Geometry check sheet. Reference: the model listing, model coordinates, mm. Face numbers are marked on the shaded views. A direction names the side the tool comes from. Round coordinates to 2 decimals unless told otherwise and drop trailing zeros. Loops run counter-clockwise (first coordinate to the right, second up) from the corner with the lowest first, then second, coordinate; pieces in that order, holes last. Notation, with made-up numbers: (-1.5, -1) -> (3.5, -1) arc R20 cw to (3.5, 14) -> close; hole circle Ø1 at (-10.5, 9.25). An arc over 180 degrees is marked (long way). Use a Markdown table: item, result. Add a question column.
Q1. Release check for a two-part mould opening along X. For the marked faces 3, 4 and 5 record: released by +X, released by -X, zero draft, split by the parting line, or undercut.
Q2. Sectioned sample at B-B, the plane z = 25.5. Enter the section's corners in (x, y).
Q3. Material ranges on L1, parallel to X at y = -10.5, z = 12; L2, parallel to Z at x = 5.5, y = -5.5; L3, parallel to Y at x = 18.25, z = 25.5, recorded low to high.
Q4. Gauge pin test, flat ends, axial feed: P1, Ø1.5, axis at x = 7.5, y = -12.5, coming from the +Z side; P2, Ø2.5, axis at x = 8.8, y = -6.51, coming from the +Z side; P3, Ø4, axis at y = -6.51, z = 25, coming from the +X side. Record the tip position at first contact, or that the pin passes through.
Q5. Sectioned sample at A-A, the plane z = 19. Enter the section's corners in (x, y).
Q6. Set-up check for the marked faces 1 and 2: record each of +Z, -Z, +X, -X, +Y, -Y from which the full face is reachable in a straight line by a thin tool's end or side.
Q7. Sectioned sample at C-C, the plane y = -8.5. Enter the section's corners in (x, z).
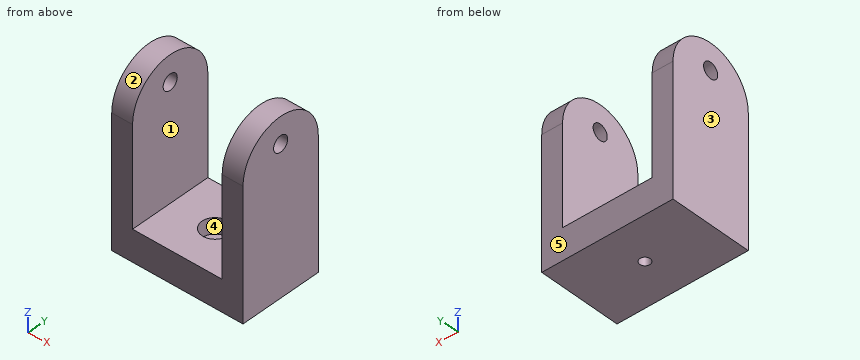
```python
from build123d import *

# Parameters (mm, degrees)
IZIM1_W                     = 25.2
IZIM1_H                     = 16
Y_KSEKLIK_EKSTR_ZYON1_DEPTH = 3
IZIM3_W                     = 4
IZIM3_H                     = 16
Y_KSEKLIK_EKSTR_ZYON2_DEPTH = 30
KES_EKSTR_ZYON3_DEPTH       = 30
IZIM5_R                     = 1.5
KES_EKSTR_ZYON4_DEPTH       = 30
IZIM6_R                     = 2.5
KES_EKSTR_ZYON5_DEPTH       = 4
IZIM7_R                     = 1
KES_EKSTR_ZYON6_DEPTH       = 15


with BuildPart() as part:
    # Çizim1 → Yükseklik-Ekstrüzyon1 (new, symmetric)
    with BuildSketch(Plane.XY):
        with Locations((8.796736324, -6.511156057)):
            Rectangle(IZIM1_W, IZIM1_H)
    extrude(amount=Y_KSEKLIK_EKSTR_ZYON1_DEPTH, both=True)

    # Çizim3 → Yükseklik-Ekstrüzyon2 (add)
    with BuildSketch(Plane.XY):
        with Locations((-1.803263676, -6.511156057)):
            Rectangle(IZIM3_W, IZIM3_H)
        with Locations((19.396736324, -6.511156057)):
            Rectangle(IZIM3_W, IZIM3_H)
    extrude(amount=Y_KSEKLIK_EKSTR_ZYON2_DEPTH)

    # Çizim4 → Kes-Ekstrüzyon3 (cut, symmetric)
    with BuildSketch(Plane(origin=(0, 0, 0), x_dir=(0, 0, -1), z_dir=(1, 0, 0))):
        with BuildLine():
            Line((-22, 1.488843943), (-31.468609906, 1.488843943))
            Line((-31.468609906, 1.488843943), (-31.468609906, -14.511156057))
            Line((-31.468609906, -14.511156057), (-22, -14.511156057))
            ThreePointArc((-22, -14.511156057), (-30, -6.511156057), (-22, 1.488843943))
        make_face()
    extrude(amount=KES_EKSTR_ZYON3_DEPTH, both=True, mode=Mode.SUBTRACT)

    # Çizim5 → Kes-Ekstrüzyon4 (cut, symmetric)
    with BuildSketch(Plane(origin=(0, 0, 0), x_dir=(0, 0, -1), z_dir=(1, 0, 0))):
        with Locations(Location((-25, -6.511156057, 0), (0, 0, 90))):
            Circle(IZIM5_R)
    extrude(amount=KES_EKSTR_ZYON4_DEPTH, both=True, mode=Mode.SUBTRACT)

    # Çizim6 → Kes-Ekstrüzyon5 (cut)
    with BuildSketch(Plane.XY):
        with Locations((8.796736324, -6.511156057)):
            Circle(IZIM6_R)
    extrude(amount=KES_EKSTR_ZYON5_DEPTH, mode=Mode.SUBTRACT)

    # Çizim7 → Kes-Ekstrüzyon6 (cut)
    with BuildSketch(Plane.XY):
        with Locations((8.796736324, -6.511156057)):
            Circle(IZIM7_R)
    extrude(amount=-KES_EKSTR_ZYON6_DEPTH, mode=Mode.SUBTRACT)


solid = part.part
```
Values:
| question | item | result |
|---|---|---|
| 1 | face 3 | released by -X |
| 1 | face 4 | undercut |
| 1 | face 5 | zero draft |
| 2 | outline | (-3.8, -13.7) -> (0.2, -13.7) -> (0.2, -7.93) -> (-3.8, -7.93) -> close; (-3.8, -5.1) -> (0.2, -5.1) -> (0.2, 0.68) -> (-3.8, 0.68) -> close; (17.4, -13.7) -> (21.4, -13.7) -> (21.4, -7.93) -> (17.4, -7.93) -> close; (17.4, -5.1) -> (21.4, -5.1) -> (21.4, 0.68) -> (17.4, 0.68) -> close |
| 3 | L1 | -3.8 to 0.2, 17.4 to 21.4 |
| 3 | L2 | -3 to 3 |
| 3 | L3 | -13.7 to -7.93, -5.1 to 0.68 |
| 4 | P1 | z = 3 |
| 4 | P2 | z = 0 |
| 4 | P3 | x = 21.4 |
| 5 | outline | (-3.8, -14.51) -> (0.2, -14.51) -> (0.2, 1.49) -> (-3.8, 1.49) -> close; (17.4, -14.51) -> (21.4, -14.51) -> (21.4, 1.49) -> (17.4, 1.49) -> close |
| 6 | face 1 | +Z, +Y, -Y |
| 6 | face 2 | +Z, +X, -X |
| 7 | outline | (-3.8, -3) -> (21.4, -3) -> (21.4, 29.75) -> (17.4, 29.75) -> (17.4, 3) -> (10.31, 3) -> (10.31, 0) -> (7.28, 0) -> (7.28, 3) -> (0.2, 3) -> (0.2, 29.75) -> (-3.8, 29.75) -> close |
